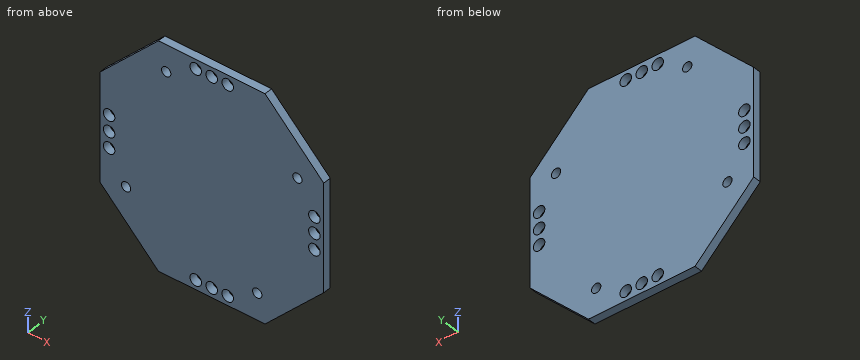
Autodesk Inventor part; units mm, degrees
ref_plane "YZ Plane" through (0, 0, 0) normal (1, 0, 0) x (0, 1, 0)
ref_plane "XZ Plane" through (0, 0, 0) normal (0, 1, 0) x (-1, 0, 0)
ref_plane "XY Plane" through (0, 0, 0) normal (0, 0, 1) x (1, 0, 0)
sketch "Esquisse1" plane through (0, 0, 0) normal (0, 1, 0) x (-1, 0, 0)
  line L0 (35, 35) -> (35, 14)
  line L1 (35, 14) -> (42, 10)
  line L2 (42, 10) -> (42, 0)
  line L3 (35, 35) -> (0, 0)
  line L4 (42, 0) -> (0, 0) construction
  line L5 (35, -35) -> (35, -14)
  line L6 (35, -14) -> (42, -10)
  line L7 (42, -10) -> (42, 0)
  line L8 (35, -35) -> (0, 0)
  line L9 (38.5, -12) -> (38.5, 12) construction
  circle A0 centre (38.5, 0) radius 2.15
  circle A1 centre (38.5, 6) radius 2.15
  circle A2 centre (38.5, -6) radius 2.15
  dimension "d0" = 90
  dimension "d1" = 70
  dimension "d4" = 6
  dimension "d11" = 6
  dimension "d16" = 4.3
  dimension "d17" = 20
  dimension "d18" = 4
  dimension "d19" = 7
extrude "Extrusion1" add sketch "Esquisse1" along normal blind 3
pattern_circular "Réseau circulaire1" count 4 over 360 about axis through (0, 0, 0) along (0, 1, 0) of "Extrusion1"
chamfer "Chanfrein1" distance 8 angle 45 4 edges at (35, 1.5, -35) (-35, 1.5, -35) (-35, 1.5, 35) (35, 1.5, 35)
ref_plane "Plan de construction3" through (-4, 0, 4) normal (0.7071, 0, 0.7071) x (0.7071, 0, -0.7071)
ref_plane "Plan de construction4" through (-4, 0, -4) normal (-0.7071, 0, 0.7071) x (0.7071, 0, 0.7071)
sketch "Esquisse15" plane through (0, 3, 0) normal (0, 1, 0) x (1, 0, 0)
  line L0 (35, -27) -> (27, -35) construction
  line L1 (35, -27) -> (35, -14) construction
  line L2 (35, -14) -> (42, -10) construction
  line L3 (42, -10) -> (42, 10) construction
  line L4 (42, 10) -> (35, 14) construction
  line L5 (35, 14) -> (35, 27) construction
  line L6 (27, 35) -> (35, 27) construction
  line L7 (27, 35) -> (14, 35) construction
  line L8 (14, 35) -> (10, 42) construction
  line L9 (10, 42) -> (-10, 42) construction
  line L10 (-10, 42) -> (-14, 35) construction
  line L11 (-14, 35) -> (-27, 35) construction
  line L12 (-35, 27) -> (-27, 35) construction
  line L13 (-35, 27) -> (-35, 14) construction
  line L14 (-35, 14) -> (-42, 10) construction
  line L15 (-42, 10) -> (-42, -10) construction
  line L16 (-42, -10) -> (-35, -14) construction
  line L17 (-35, -14) -> (-35, -27) construction
  line L18 (-27, -35) -> (-35, -27) construction
  line L19 (-27, -35) -> (-14, -35) construction
  line L20 (-14, -35) -> (-10, -42) construction
  line L21 (-10, -42) -> (10, -42) construction
  line L22 (10, -42) -> (14, -35) construction
  line L23 (14, -35) -> (27, -35) construction
  circle A0 centre (0, -38.5) radius 2.15 construction
  circle A1 centre (6, -38.5) radius 2.15 construction
  circle A2 centre (-6, -38.5) radius 2.15 construction
  circle A3 centre (38.5, -6) radius 2.15 construction
  circle A4 centre (38.5, 6) radius 2.15 construction
  circle A5 centre (38.5, 0) radius 2.15 construction
  circle A6 centre (6, 38.5) radius 2.15 construction
  circle A7 centre (-6, 38.5) radius 2.15 construction
  circle A8 centre (0, 38.5) radius 2.15 construction
  circle A9 centre (-38.5, 6) radius 2.15 construction
  circle A10 centre (-38.5, -6) radius 2.15 construction
  circle A11 centre (-38.5, 0) radius 2.15 construction
  line L24 (10, 42) -> (20, 42)
  line L25 (20, 42) -> (42, 20)
  line L26 (42, -10) -> (42, 10)
  line L27 (42, 20) -> (42, 10)
  line L28 (27, 35) -> (35, 27)
  line L29 (0, 0) -> (42, 10)
  line L30 (10, 42) -> (0, 0)
  line L31 (10, 42) -> (-10, 42)
extrude "Extrusion13" add sketch "Esquisse15" against normal blind 3
pattern_circular "Réseau circulaire7" count 4 over 360 about axis through (0, 0, 0) along (0, 1, 0) of "Extrusion13"
sketch "Esquisse9" plane through (0, 0, 0) normal (0, -1, 0) x (1, 0, 0)
  line L0 (0, 0) -> (21.8388, 21.8388) construction
  line L1 (0, 0) -> (66.7346, 0) construction
  line L2 (0, 0) -> (0, 22.6965) construction
  line L3 (31.4289, 0) -> (31.4289, 10)
  line L4 (31.4289, 10) -> (38.5, 17.0711)
  line L5 (38.5, 17.0711) -> (27.7855, 27.7855)
  line L6 (0, 31.4289) -> (10, 31.4289)
  line L7 (10, 31.4289) -> (17.0711, 38.5)
  line L8 (17.0711, 38.5) -> (27.7855, 27.7855)
  line L9 (38.5, -17.0711) -> (27.7855, -27.7855)
  line L10 (31.4289, -10) -> (38.5, -17.0711)
  line L11 (31.4289, 0) -> (31.4289, -10)
  line L12 (17.0711, -38.5) -> (27.7855, -27.7855)
  line L13 (10, -31.4289) -> (17.0711, -38.5)
  line L14 (0, -31.4289) -> (10, -31.4289)
  line L15 (-31.4289, 0) -> (-31.4289, -10)
  line L16 (-31.4289, -10) -> (-38.5, -17.0711)
  line L17 (-38.5, -17.0711) -> (-27.7855, -27.7855)
  line L18 (-17.0711, -38.5) -> (-27.7855, -27.7855)
  line L19 (0, -31.4289) -> (-10, -31.4289)
  line L20 (-10, -31.4289) -> (-17.0711, -38.5)
  line L21 (0, 0) -> (-66.7346, 0) construction
  line L22 (-31.4289, 0) -> (-31.4289, 10)
  line L23 (-31.4289, 10) -> (-38.5, 17.0711)
  line L24 (0, 31.4289) -> (-10, 31.4289)
  line L25 (0, 0) -> (-21.8388, 21.8388) construction
  line L26 (-10, 31.4289) -> (-17.0711, 38.5)
  line L27 (-17.0711, 38.5) -> (-27.7855, 27.7855)
  line L28 (-38.5, 17.0711) -> (-27.7855, 27.7855)
  line L29 (27.432, 27.432) -> (37.7929, 17.0711)
  line L30 (37.7929, 17.0711) -> (30.9289, 10.2071)
  line L31 (30.9289, 10.2071) -> (30.9289, 0)
  line L32 (30.9289, 0) -> (30.9289, -10.2071)
  line L33 (30.9289, -10.2071) -> (37.7929, -17.0711)
  line L34 (37.7929, -17.0711) -> (27.432, -27.432)
  line L35 (27.432, -27.432) -> (17.0711, -37.7929)
  line L36 (17.0711, -37.7929) -> (10.2071, -30.9289)
  line L37 (10.2071, -30.9289) -> (0, -30.9289)
  line L38 (0, -30.9289) -> (-10.2071, -30.9289)
  line L39 (-10.2071, -30.9289) -> (-17.0711, -37.7929)
  line L40 (-17.0711, -37.7929) -> (-27.432, -27.432)
  line L41 (-27.432, -27.432) -> (-37.7929, -17.0711)
  line L42 (-37.7929, -17.0711) -> (-30.9289, -10.2071)
  line L43 (-30.9289, -10.2071) -> (-30.9289, 0)
  line L44 (-30.9289, 0) -> (-30.9289, 10.2071)
  line L45 (-30.9289, 10.2071) -> (-37.7929, 17.0711)
  line L46 (-37.7929, 17.0711) -> (-27.432, 27.432)
  line L47 (-27.432, 27.432) -> (-17.0711, 37.7929)
  line L48 (-17.0711, 37.7929) -> (-10.2071, 30.9289)
  line L49 (-10.2071, 30.9289) -> (0, 30.9289)
  line L50 (0, 30.9289) -> (10.2071, 30.9289)
  line L51 (10.2071, 30.9289) -> (17.0711, 37.7929)
  line L52 (17.0711, 37.7929) -> (27.432, 27.432)
  dimension "d67" = 45
  dimension "d68" = 10
  dimension "d69" = 10
  dimension "d70" = 38.5
  dimension "d71" = 77
  dimension "d86" = 0.5
extrude "Extrusion9" cut sketch "Esquisse9" against normal through all contours L29 L30 L31 L32 L33 L34 L35 L36 L37 L38 L39 L40 L41 L42 L43 L44 L45 L46 L47 L48 L49 L50 L51 L52
sketch "Esquisse12" plane through (0, 3, 0) normal (0, 1, 0) x (1, 0, 0)
  line L0 (-10, -31.4289) -> (-17.0711, -38.5)
  line L1 (-17.0711, -38.5) -> (-27.7855, -27.7855)
  line L2 (-31.4289, -10) -> (-38.5, -17.0711)
  line L3 (-38.5, -17.0711) -> (-27.7855, -27.7855)
  line L4 (-10, -31.4289) -> (-15.6569, -25.7721)
  line L5 (-15.6569, -25.7721) -> (-22.7279, -32.8431)
  circle A0 centre (-17.0711, -32.136) radius 1.75
  line L6 (-10, -31.4289) -> (-17.0711, -38.5)
  line L7 (-17.0711, -38.5) -> (-22.7279, -32.8431)
  line L8 (31.4289, -10) -> (25.7721, -15.6569)
  line L9 (25.7721, -15.6569) -> (32.8431, -22.7279)
  circle A1 centre (32.136, -17.0711) radius 1.75
  line L10 (31.4289, -10) -> (38.5, -17.0711)
  line L11 (38.5, -17.0711) -> (32.8431, -22.7279)
  line L12 (10, 31.4289) -> (15.6569, 25.7721)
  line L13 (15.6569, 25.7721) -> (22.7279, 32.8431)
  circle A2 centre (17.0711, 32.136) radius 1.75
  line L14 (10, 31.4289) -> (17.0711, 38.5)
  line L15 (17.0711, 38.5) -> (22.7279, 32.8431)
  line L16 (-31.4289, 10) -> (-25.7721, 15.6569)
  line L17 (-25.7721, 15.6569) -> (-32.8431, 22.7279)
  circle A3 centre (-32.136, 17.0711) radius 1.75
  line L18 (-31.4289, 10) -> (-38.5, 17.0711)
  line L19 (-38.5, 17.0711) -> (-32.8431, 22.7279)
  point P0 (0, 0)
  dimension "d32" = 8
  dimension "d89" = 4.5
  dimension "d90" = 4.5
  dimension "d91" = 3.5
  dimension "d94" = 360
  dimension "d98" = 8
extrude "Extrusion10" add sketch "Esquisse12" against normal blind 3
sketch "Esquisse14" plane through (0, 3, 0) normal (0, 1, 0) x (1, 0, 0)
  line L0 (20, 42) -> (42, 20)
  line L1 (-42, 20) -> (-20, 42)
  line L2 (-20, -42) -> (-42, -20)
  line L3 (42, -20) -> (20, -42)
  circle A0 centre (17.0711, 32.136) radius 1.75
  circle A1 centre (-17.0711, -32.136) radius 1.75
  circle A2 centre (32.136, -17.0711) radius 1.75
  circle A3 centre (-32.136, 17.0711) radius 1.75
  line L4 (22.3744, 32.4896) -> (37.7929, 17.0711)
  line L5 (37.7929, 17.0711) -> (30.9289, 10.2071)
  line L6 (30.9289, 10.2071) -> (30.9289, -10.2071)
  line L7 (30.9289, -10.2071) -> (31.0754, -10.3536)
  line L8 (25.7721, -15.6569) -> (31.0754, -10.3536)
  line L9 (32.4896, -22.3744) -> (25.7721, -15.6569)
  line L10 (32.4896, -22.3744) -> (17.0711, -37.7929)
  line L11 (17.0711, -37.7929) -> (10.2071, -30.9289)
  line L12 (10.2071, -30.9289) -> (-10.2071, -30.9289)
  line L13 (-10.2071, -30.9289) -> (-10.3536, -31.0754)
  line L14 (-10.3536, -31.0754) -> (-15.6569, -25.7721)
  line L15 (-15.6569, -25.7721) -> (-22.3744, -32.4896)
  line L16 (-22.3744, -32.4896) -> (-37.7929, -17.0711)
  line L17 (-37.7929, -17.0711) -> (-30.9289, -10.2071)
  line L18 (-30.9289, -10.2071) -> (-30.9289, 10.2071)
  line L19 (-30.9289, 10.2071) -> (-31.0754, 10.3536)
  line L20 (-25.7721, 15.6569) -> (-31.0754, 10.3536)
  line L21 (-32.4896, 22.3744) -> (-25.7721, 15.6569)
  line L22 (-32.4896, 22.3744) -> (-17.0711, 37.7929)
  line L23 (-17.0711, 37.7929) -> (-10.2071, 30.9289)
  line L24 (-10.2071, 30.9289) -> (10.2071, 30.9289)
  line L25 (10.2071, 30.9289) -> (10.3536, 31.0754)
  line L26 (15.6569, 25.7721) -> (10.3536, 31.0754)
  line L27 (22.3744, 32.4896) -> (15.6569, 25.7721)
  circle A4 centre (38.5, 0) radius 2.15
  circle A5 centre (38.5, 6) radius 2.15
  circle A6 centre (38.5, -6) radius 2.15
  circle A7 centre (-6, -38.5) radius 2.15
  circle A8 centre (6, -38.5) radius 2.15
  circle A9 centre (0, -38.5) radius 2.15
  circle A10 centre (-38.5, 0) radius 2.15
  circle A11 centre (-38.5, -6) radius 2.15
  circle A12 centre (-38.5, 6) radius 2.15
  circle A13 centre (0, 38.5) radius 2.15
  circle A14 centre (-6, 38.5) radius 2.15
  circle A15 centre (6, 38.5) radius 2.15
  line L28 (42, 20) -> (42, -20)
  line L29 (-20, 42) -> (20, 42)
  line L30 (-42, -20) -> (-42, 20)
  line L31 (20, -42) -> (-20, -42)
  point P0 (0, 0)
extrude "Extrusion12" add sketch "Esquisse14" against normal blind 3 contours L4 L5 L6 L7 L8 L9 L10 L11 L12 L13 L14 L15 L16 L17 L18 L19 L20 L21 L22 L23 L24 L25 L26 L27
properties part number "bottom"
Geometry: final body of the model. Coordinates: model frame, mm. Give positions to 0.01 mm unless a question says otherwise; leave off trailing zeros. Write each loop counter-clockwise with the first axis right and the second up, starting at its lowest first coordinate (ties: lowest second). Pieces come first, ordered by that corner, then holes. Notation, with made-up numbers: (67, 13) -> (126, 13) arc R24 ccw to (126, 41) -> close; hole circle Ø7 at (-25, 60). An arc over 180 degrees is marked (long way). Answer in a Markdown table with one row per item.
(1) Section query C-C on z = 38.5. Return loops of the section in (x, y).
Answers below:
| item | result |
|---|---|
| outline | (-23.5, 0) -> (-8.15, 0) -> (-8.15, 3) -> (-23.5, 3) -> close; (-3.85, 0) -> (-2.15, 0) -> (-2.15, 3) -> (-3.85, 3) -> close; (2.15, 0) -> (3.85, 0) -> (3.85, 3) -> (2.15, 3) -> close; (8.15, 0) -> (23.5, 0) -> (23.5, 3) -> (8.15, 3) -> close |
(2) Section query A-A on x = 0. Return loops of the section in (y, z).
Answers below:
| item | result |
|---|---|
| outline | (0, -42) -> (3, -42) -> (3, -40.65) -> (0, -40.65) -> close; (0, -36.35) -> (3, -36.35) -> (3, 36.35) -> (0, 36.35) -> close; (0, 40.65) -> (3, 40.65) -> (3, 42) -> (0, 42) -> close |
(3) Section query D-D on y = 1.55. State how many separate pieces and enclosed holes the cut face has, then the cut area to 3 significant figures.
Answers below:
| item | result |
|---|---|
| separate pieces | 1 |
| enclosed holes | 16 |
| area | 5,880 mm^2 |
(4) Section query B-B on z = -6. Return loops of the section in (x, y).
Answers below:
| item | result |
|---|---|
| outline | (-42, 0) -> (-40.65, 0) -> (-40.65, 3) -> (-42, 3) -> close; (-36.35, 0) -> (36.35, 0) -> (36.35, 3) -> (-36.35, 3) -> close; (40.65, 0) -> (42, 0) -> (42, 3) -> (40.65, 3) -> close |
(5) Pin query (flat end, axial travel): pin 1 (3 mm diameter, centred on x = -17.07, z = 32.14, fed in from +Y); pin 2 (5.5 mm diameter, centred on x = -38.5, z = -6, fed in from -Y). Return the tip coordinate at first contact, or that it passes through.
Answers below:
| item | result |
|---|---|
| pin 1 | through |
| pin 2 | y = 0 |
(6) Ray query, line 1 along X through (y, z) = (2.3, -38.5); line 2 along X through (y, z) = (0.2, -37). Return the intervals inside material, ascending. Write a range as [from, to].
Answers below:
| item | result |
|---|---|
| line 1 | [-23.5, -8.15], [-3.85, -2.15], [2.15, 3.85], [8.15, 23.5] |
| line 2 | [-25, -7.54], [-4.46, -1.54], [1.54, 4.46], [7.54, 25] |
